```python
from build123d import *

# Parameters (mm, degrees)
THICKEN1_DEPTH     = 215
SKETCH5_W          = 2293.9698
SKETCH5_H          = 1307.808
CUT_EXTRUDE1_DEPTH = 1837.971398424


# Read off the part's stored shape, not the designer's step: Thicken1
with BuildPart() as part:
    # Thicken1 outline → Thicken1 (new body)
    with BuildSketch(Plane(origin=(0, 0, 0), x_dir=(1, 0, 0), z_dir=(0, 1, 0))):
        with BuildLine():
            Line((35.85, -1307.808), (1022.0118, -1307.808))
            Line((1022.0118, -1307.808), (1022.0118, 1307.808))
            Line((1022.0118, 1307.808), (35.85, 1307.808))
            ThreePointArc((35.85, 1307.808), (-1271.958, 0), (35.85, -1307.808))
        make_face()
        with BuildLine():
            Line((305, 0), (35.85, -35.85))
            ThreePointArc((35.85, -35.85), (0, 0), (35.85, 35.85))
            Line((35.85, 35.85), (305, 0))
        make_face(mode=Mode.SUBTRACT)
    extrude(amount=THICKEN1_DEPTH)

    # Sketch5 → Cut-Extrude1 (cut, through all)
    with BuildSketch(Plane(origin=(0, 215, 0), x_dir=(1, 0, 0), z_dir=(0, 1, 0))):
        with Locations((-124.9731, 653.904)):
            Rectangle(SKETCH5_W, SKETCH5_H)
    extrude(amount=-CUT_EXTRUDE1_DEPTH, mode=Mode.SUBTRACT)


solid = part.part
```
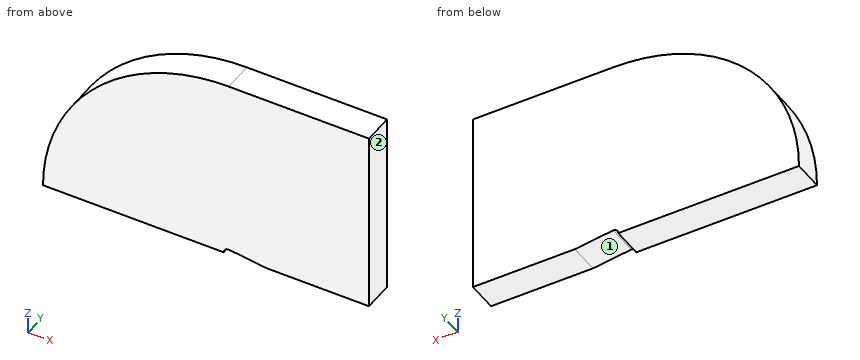
Design review of the part built by this model. Coordinates are the model's own, in mm. Face numbers are marked on the shaded views. A direction names the side the tool comes from. Coordinates: 2 decimals unless noted, no trailing zeros. Order: outer loops, then holes, each group sorted by start corner. A loop starts at its lowest first (then second) coordinate and runs counter-clockwise, first axis right, second up. Notation, with made-up numbers: M 56.5,20.25 L 96.5,20.25 A17 cw 96.5,34.25 Z; hole C 58.5,-0.5 d5. An arc over 180 degrees is marked long. Answer as a JSON object with one key per item and string values. Group by question number.
1) For pin 1 (10 mm diameter, centred on x = -847.5, z = 550, fed in from -Y); pin 2 (6 mm diameter, centred on y = 86, z = 558.5, fed in from -X); pin 3 (6 mm diameter, centred on x = -668.5, y = 127.5, fed in from +Z); pin 4 (2 mm diameter, centred on y = 37.5, z = 601, fed in from -X), all flat-tipped, find the tip position at first contact; note any pin that passes through.
2) Add section A-A, the plane y = 153. Write out the cut boundary in (x, z), then the cut area to 3 significant figures.
3) Add section B-B, the plane z = 829. Write out the cut boundary in (x, y).
4) Tool access review of the marked faces 1 and 2: name each direction out of +Z, -Z, +X, -X, +Y, -Y from which nothing blocks a thin tool from reaching the whole face with its end or side.
5) Wall thickness on L1, parallel to Z at x = -238.5, y = 95.5; L2, parallel to X at y = 81, z = 273.5; L3, parallel to X at y = 41, z = 232: over which ranges is each line inside the solid? List them lowest first.
6) Add section C-C, the plane z = 1030.5. Write out the cut boundary in (x, y), then the cut area to 3 significant figures.
Computed values:
{
 "1": {"pin 1": "stops at y = 0", "pin 2": "stops at x = -1148.12", "pin 3": "stops at z = 1103.84", "pin 4": "stops at x = -1126.2"},
 "2": {"outline": "M -1271.96,0 L 0,0 A35.85 cw 35.85,35.85 L 305,0 L 1022.01,0 L 1022.01,1307.81 L 35.85,1307.81 A1307.81 ccw Z", "area": "2,630,000 mm^2"},
 "3": {"outline": "M -975.64,0 L 1022.01,0 L 1022.01,215 L -975.64,215 Z"},
 "4": {"face 1": "-Z, +Y, -Y", "face 2": "+Z, -Z, +X, +Y, -Y"},
 "5": {"L1": "z = 0 to 1278.71", "L2": "x = -1243.04 to 1022.01", "L3": "x = -1251.22 to 1022.01"},
 "6": {"outline": "M -769.4,0 L 1022.01,0 L 1022.01,215 L -769.4,215 Z", "area": "385,000 mm^2"}
}
